Design review of the part built by this model. Coordinates are the model's own, in mm. Coordinates: 2 decimals unless noted, no trailing zeros. Write each loop counter-clockwise with the first axis right and the second up, starting at its lowest first coordinate (ties: lowest second). Pieces come first, ordered by that corner, then holes.
Q1. For probe 1 along Z at (x, y) = (0, -0.25); probe 2 along Z at (x, y) = (-1.25, -1.5); probe 3 along X at (y, z) = (-3, -2.25), list the stretches that pass through material, from the lowest coordinate up.
Q2. Take a section at C-C (z = -4). Give the boundary of the cut face in (x, y), and give its area (3 significant figures).
Q3. Take a section at D-D (x = 3.25). Give the boundary of the cut face in (y, z), and give its area (3 significant figures).
Q4. Insertion check: pin 1 (1 mm diameter, centred on y = -3.5, z = 3, fed in from +X); pin 2 (1.5 mm diameter, centred on x = -3, z = 1.5, fed in from -Y); pin 3 (3 mm diameter, centred on x = 3.5, z = 2, fed in from +Y). Each pin has a flat end and moves straight along its axis. Give the tip position at first contact, or say it passes through.
Q5. Take a section at A-A (x = 0). Give the boundary of the cut face in (y, z), and give its area (3 significant figures).
Q6. Take a section at B-B (y = 4). Give the boundary of the cut face in (x, z), and give its area (3 significant figures).
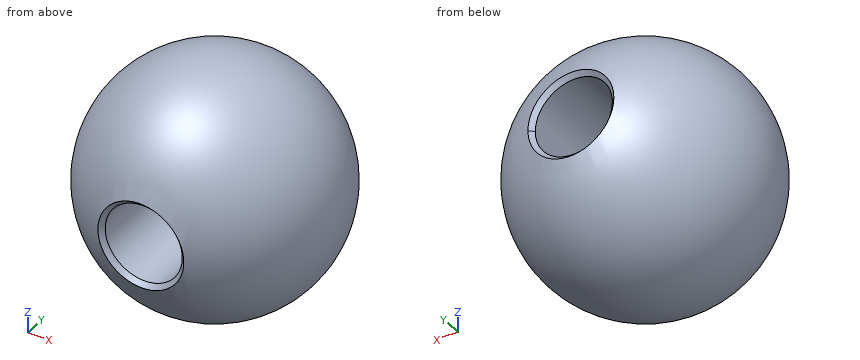
```python
from build123d import *

# Parameters (mm, degrees)
M3_CLEARANCE_HOLE1_D = 3.2
CHAMFER1_SIZE        = 0.25


with BuildPart() as part:
    # Sketch2 → Revolve1 (revolve)
    with BuildSketch(Plane.XY):
        with BuildLine():
            Line((-5, 0), (5, 0))
            ThreePointArc((5, 0), (0, 5), (-5, 0))
        make_face()
    revolve(axis=Axis((-5, 0, 0), (1, 0, 0)))

    # M3 Clearance Hole1 (through all)
    with Locations(Plane(origin=(0, 5, 0), x_dir=(1, 0, 0), z_dir=(0, 1, 0))):
        with Locations((0, 0)):
            Hole(M3_CLEARANCE_HOLE1_D / 2)

    # Chamfer1
    # the kernel refuses this chamfer: 0.25, 0.197251491 mm, written as the material it takes off along each edge
    with BuildSketch(Plane(origin=(-3e-09, -4.737087713, 0), x_dir=(-1.0, 0, -1.7241398847038223e-10), z_dir=(-1.7241398847038223e-10, 0, 1.0))) as chamfer1_piece_1:
        with BuildLine():
            Line((1.783867045, -0.066132952), (1.600000003, -0.249999994))
            Line((1.600000003, -0.249999994), (1.599999997, 0))
            ThreePointArc((1.599999997, 0), (1.69425958, -0.032889111), (1.783867045, -0.066132952))
        make_face()
    revolve(axis=Axis((-3e-09, -4.737087713, 0), (0, -1, 0)), mode=Mode.SUBTRACT)
    with BuildSketch(Plane(origin=(0, 4.737087713, 5e-09), x_dir=(-1.0, 0, -2.962106121087604e-09), z_dir=(-2.962106121087604e-09, 0, 1.0))) as chamfer1_piece_2:
        with BuildLine():
            Line((1.783867047, 0.066132952), (1.600000005, 0.249999995))
            Line((1.600000005, 0.249999995), (1.6, 0))
            ThreePointArc((1.6, 0), (1.694259582, 0.032889111), (1.783867047, 0.066132952))
        make_face()
    revolve(axis=Axis((0, 4.737087713, 5e-09), (0, -1, 0)), revolution_arc=179.999999661, mode=Mode.SUBTRACT)
    with BuildSketch(Plane(origin=(0, 4.737087713, 0), x_dir=(1.0, 0, -6.014235446318052e-11), z_dir=(-6.014235446318052e-11, -1.2821909266166277e-15, -1.0))) as chamfer1_piece_3:
        with BuildLine():
            Line((1.783867046, 0.066132954), (1.6, CHAMFER1_SIZE))
            Line((1.6, CHAMFER1_SIZE), (1.6, 0))
            ThreePointArc((1.6, 0), (1.694259582, 0.032889113), (1.783867046, 0.066132954))
        make_face()
    revolve(axis=Axis((0, 4.737087713, 0), (0, -1, 0)), revolution_arc=180.000000007, mode=Mode.SUBTRACT)


solid = part.part
```
Response:
1. probe 1: z = -4.99 to -1.6, 1.6 to 4.99
1. probe 2: z = -4.6 to -1, 1 to 4.6
1. probe 3: x = -3.31 to 3.31
2. outline: circle Ø6 at (0, 0)
2. area: 28.3 mm2
3. outline: circle Ø7.6 at (0, 0)
3. area: 45.4 mm2
4. pin 1: stops at x = 2.85
4. pin 2: stops at y = -4.27
4. pin 3: stops at y = 4.31
5. outline: (-4.67, -1.78) arc R5 ccw to (4.67, -1.78) - (4.49, -1.6) - (-4.49, -1.6) - close; (-4.67, 1.78) - (-4.49, 1.6) - (4.49, 1.6) - (4.67, 1.78) arc R5 ccw to start
5. area: 47.0 mm2
6. outline: circle Ø6 at (0, 0); hole circle Ø3.2 at (0, 0)
6. area: 20.2 mm2
